Geometry check sheet. Reference: the model listing, model coordinates, mm. A direction names the side the tool comes from. Round coordinates to 2 decimals unless told otherwise and drop trailing zeros. Write each loop counter-clockwise with the first axis right and the second up, starting at its lowest first coordinate (ties: lowest second). Pieces come first, ordered by that corner, then holes. Notation, with made-up numbers: M 42,81.25 L 63,81.25 A17 ccw 63,110.25 Z; hole C 56,47.25 d7. An arc over 180 degrees is marked long. Answer in a Markdown table with one row per item. Add a question column.
from build123d import *

# Parameters (mm, degrees)
BOSS_EXTRUDE2_DEPTH      = 304.8
BOSS_EXTRUDE2_DEPTH_BACK = 1286.002


with BuildPart() as part:
    # Sketch1 → Boss-Extrude2 (new, two sides: drawn at the far end of the back side and taken through both)
    with BuildSketch(Plane.XY.offset(-BOSS_EXTRUDE2_DEPTH_BACK)):
        with BuildLine():
            Line((0, -9.525), (0, -923.925))
            Line((0, -923.925), (-243.93812726, -923.925))
            Line((-243.93812726, -923.925), (-243.93812726, -243.93812726))
            Line((-243.93812726, -243.93812726), (-923.925, -243.93812726))
            Line((-923.925, -243.93812726), (-923.925, 0))
            Line((-923.925, 0), (-9.525, 0))
            ThreePointArc((-9.525, 0), (-2.789807909, -2.789807909), (0, -9.525))
        make_face()
    extrude(amount=BOSS_EXTRUDE2_DEPTH + BOSS_EXTRUDE2_DEPTH_BACK)


solid = part.part
Item 1: Section check A-A, the plane z = -13.5. Record the boundary of the cut face in (x, y) (3 decimals).
Item 2: Scan line: probe 1 along X at (y, z) = (-801, -378). Record every from-to range of solid material in increasing order. Write a range as from..to.
Item 3: Access from +Z, -Z, +X, -X, +Y, -Y to the whole of each face (thin tool, end or side, straight path). Record for faces 1 (the flat face through (-579, -243.938, -502)), 2 (the flat face through (-120, -923.925, -502)).
Item 4: Gauge pin test, flat end, axial feed: pin 1 Ø3 at (x, z) = (-503, -404) entering from -Y. Record the tip position at first contact, or that the pin passes through.
Item 5: Section check B-B, the plane x = -673. Record the boundary of the cut face in (y, z).
Result sheet:
| question | item | result |
|---|---|---|
| 1 | outline | M -923.925,-243.938 L -243.938,-243.938 L -243.938,-923.925 L 0,-923.925 L 0,-9.525 A9.525 ccw -9.525,0 L -923.925,0 Z |
| 2 | probe 1 | x = -243.94..0 |
| 3 | face 1 | +Z, -Z, -X, -Y |
| 3 | face 2 | +Z, -Z, +X, -X, -Y |
| 4 | pin 1 | stops at y = -243.94 |
| 5 | outline | M -243.94,-1286 L 0,-1286 L 0,304.8 L -243.94,304.8 Z |
